Part model, mm, in its own coordinate system. A direction names the side the tool comes from. Round coordinates to 2 decimals unless told otherwise and drop trailing zeros. Return JSON: item names as keys, results as strings. Group by question number.
(1) Tool access for faces 4 (the flat face through (2, -5, 3)), 5 (the flat face through (-0.1, -2.2, 2)), 6 (the flat face through (-0.1, -2.2, -2)): list every direction of +Z, -Z, +X, -X, +Y, -Y with a clear straight run to the whole face (end or side of a thin tool).
(2) Drop a flat-ended pin along its axis: pin 1 Ø2.5 at (x, y) = (0, 0) entering from -Z. Give the stop position or say it passes through.
(3) Mould opens along X. For faces 1 (the cylindrical face through (0, -2, 0)), 2 (the cylindrical face through (-1.08, -4.88, -2.51)), 3 (the flat face through (2, -5, -3)) say: +X half, -X half, draft (parallel to the pull), parting line (faces both ways), or undercut.
from build123d import *
from build123d.topology import SkipClean

# Parameters (mm, degrees)
CUT_EXTRUDE_START   = 3
SKETCH_2_R          = 9.058655207
CUT_EXTRUDE_1_DEPTH = 10
CUT_EXTRUDE_START_2 = -3
SKETCH_2_2_R        = 9.058655207
CUT_EXTRUDE_2_DEPTH = 10
SKETCH_3_R          = 5
CUT_EXTRUDE_3_DEPTH = 1
SKETCH_4_R          = 2
CUT_EXTRUDE_4_DEPTH = 5


with BuildPart() as part:
    # 草图1 → 旋转3 (revolve)
    with SkipClean():  # the faces are left unmerged after this step: merging them gives an invalid solid
        with BuildSketch(Plane.XY):
            with BuildLine():
                ThreePointArc((8, 0), (5.656854249, 5.656854249), (0, 8))
                Line((0, 8), (0, -8))
                ThreePointArc((0, -8), (5.656854249, -5.656854249), (8, 0))
            make_face()
            with BuildLine():
                Line((0, -8), (0, 8))
                ThreePointArc((0, 8), (-8, 0), (0, -8))
            make_face()
        revolve(axis=Axis((0, 8, 0), (0, -1, 0)))

    # 草图2 → 切除-拉伸1 (cut)
    with SkipClean():  # the faces are left unmerged after this step: merging them gives an invalid solid
        with BuildSketch(Plane.XY.offset(CUT_EXTRUDE_START)):
            Circle(SKETCH_2_R)
        extrude(amount=CUT_EXTRUDE_1_DEPTH, mode=Mode.SUBTRACT)

    # 草图2<2> → 切除-拉伸2 (cut)
    with SkipClean():  # the faces are left unmerged after this step: merging them gives an invalid solid
        with BuildSketch(Plane.XY.offset(CUT_EXTRUDE_START_2)):
            Circle(SKETCH_2_2_R)
        extrude(amount=-CUT_EXTRUDE_2_DEPTH, mode=Mode.SUBTRACT)

    # 草图3 → 切除-拉伸3 (cut)
    with SkipClean():  # the faces are left unmerged after this step: merging them gives an invalid solid
        with BuildSketch(Plane.XY.offset(3)):
            Circle(SKETCH_3_R)
        cut_extrude_3 = extrude(amount=-CUT_EXTRUDE_3_DEPTH, mode=Mode.SUBTRACT)

    # 镜向1: 切除-拉伸3 across plane
    with SkipClean():  # the faces are left unmerged after this step: merging them gives an invalid solid
        add(cut_extrude_3.mirror(Plane.XY), mode=Mode.SUBTRACT)

    # 草图4 → 切除-拉伸4 (cut)
    with SkipClean():  # the faces are left unmerged after this step: merging them gives an invalid solid
        with BuildSketch(Plane.XY.offset(2)):
            Circle(SKETCH_4_R)
        extrude(amount=-CUT_EXTRUDE_4_DEPTH, mode=Mode.SUBTRACT)


solid = part.part
Computed values:
{
 "1": {"face 4": "+Z, +X, -X, +Y, -Y", "face 5": "+Z", "face 6": "-Z"},
 "2": {"pin 1": "through"},
 "3": {"face 1": "undercut", "face 2": "undercut", "face 3": "draft"}
}
